Verification items for this drawing (mm, ordinates from the low corner). Round coordinates to 2 decimals unless told otherwise and drop trailing zeros. Order: outer loops, then holes, each group sorted by start corner. A loop starts at its lowest first (then second) coordinate and runs counter-clockwise, first axis right, second up.
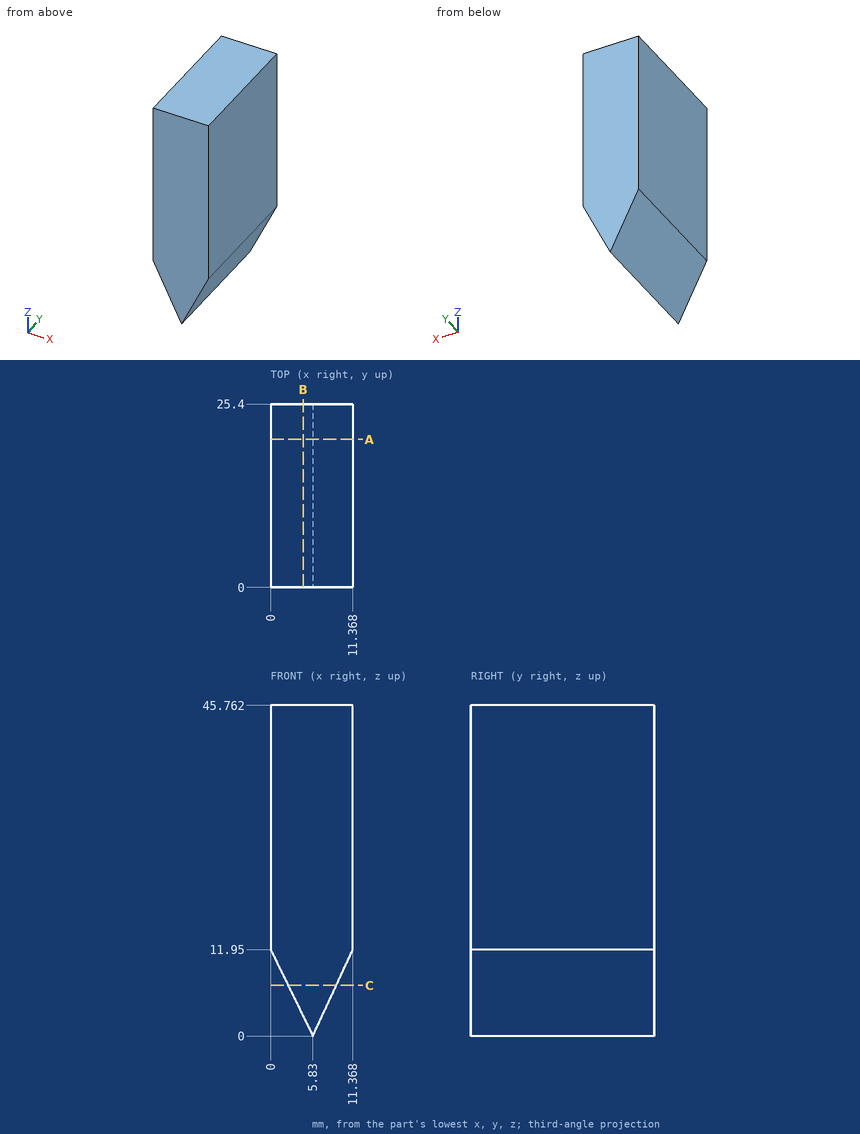
Item 1: Scan lines: line 1 along Z through (x, y) = (8, 23) (1 decimal); line 2 along X through (y, z) = (23.75, 4) (1 decimal); line 3 along Z through (x, y) = (1.5, 1.75) (1 decimal). Record each from-to range of solid material in increasing order.
Answer:
line 1: z = 4.7 to 45.8
line 2: x = 3.9 to 7.7
line 3: z = 8.9 to 45.8
Item 2: Sectioned sample at A-A (y = 20.5). Record the cut outline in (x, z).
Answer:
outline: (0, 11.95) - (5.83, 0) - (11.37, 11.95) - (11.37, 45.76) - (0, 45.76) - close
Item 3: Sectioned sample at B-B (x = 4.5). Record the cut outline in (y, z) (1 decimal).
Answer:
outline: (0, 2.7) - (25.4, 2.7) - (25.4, 45.8) - (0, 45.8) - close
Item 4: Go/stop test with flat-tipped pins: P1, Ø4, axis at y = 17, z = 41, coming from the -X side; P2, Ø4, axis at x = 9, y = 8, coming from the -Z side (1 decimal); P3, Ø1.5, axis at y = 16.5, z = 11, coming from the +X side (1 decimal). Record where each tip stops, or that it passes through.
Answer:
P1: stops at x = 0
P2: stops at z = 2.5
P3: stops at x = 11.3
Item 5: Sectioned sample at C-C (z = 7). Record the cut outline in (x, y) (1 decimal).
Answer:
outline: (2.4, 0) - (9.1, 0) - (9.1, 25.4) - (2.4, 25.4) - close
